Input: dimensioned drawing with shaded views. Units: mm. Origin: part minimum x, y, z. A direction names the side the tool comes from. Round coordinates to 2 decimals unless told otherwise and drop trailing zeros. Loops run counter-clockwise (first coordinate to the right, second up) from the corner with the lowest first, then second, coordinate; pieces in that order, holes last. Notation, with made-up numbers: (-8, -7.75) - (3, -7.75) arc R12 ccw to (3, -3.75) - close; hole circle Ø3 at (40.25, -34). An arc over 180 degrees is marked (long way). One line per question, with ' | ' between items. Start each with the question number.
Item 1: Section D-D, the plane z = 86. Return loops of the section in (x, y).
Item 2: First-contact query: pin 1 (12 mm diameter, centred on y = 122, z = 266, fed in from -X); pin 2 (3 mm diameter, centred on x = 233.5, z = 801.5, fed in from -Y); pin 3 (10 mm diameter, centred on x = 418, z = 441.5, fed in from +Y). Flat tips, straight axial feed; report the tip coordinate or a pass-through.
Item 3: Section B-B, the plane z = 562. Return loops of the section in (x, y).
Item 4: Section C-C, the plane x = 327.5. Return loops of the section in (y, z), plus the area to 3 significant figures.
Item 5: Material intervals for line 1 along Z through (x, y) = (676, 86); line 2 along Y through (x, z) = (394, 626.5); line 3 along Y through (x, z) = (71.5, 714), sorted ascending.
Item 6: Section A-A, the plane y = 75. Return loops of the section in (x, z), plus the area to 3 significant figures.
Item 7: Set-up query: the marked faces 1, 2 and 3. Return all of +Z, -Z, +X, -X, +Y, -Y with unobstructed straight access to the full face (end or side cutting, diameter ignored); none if empty.
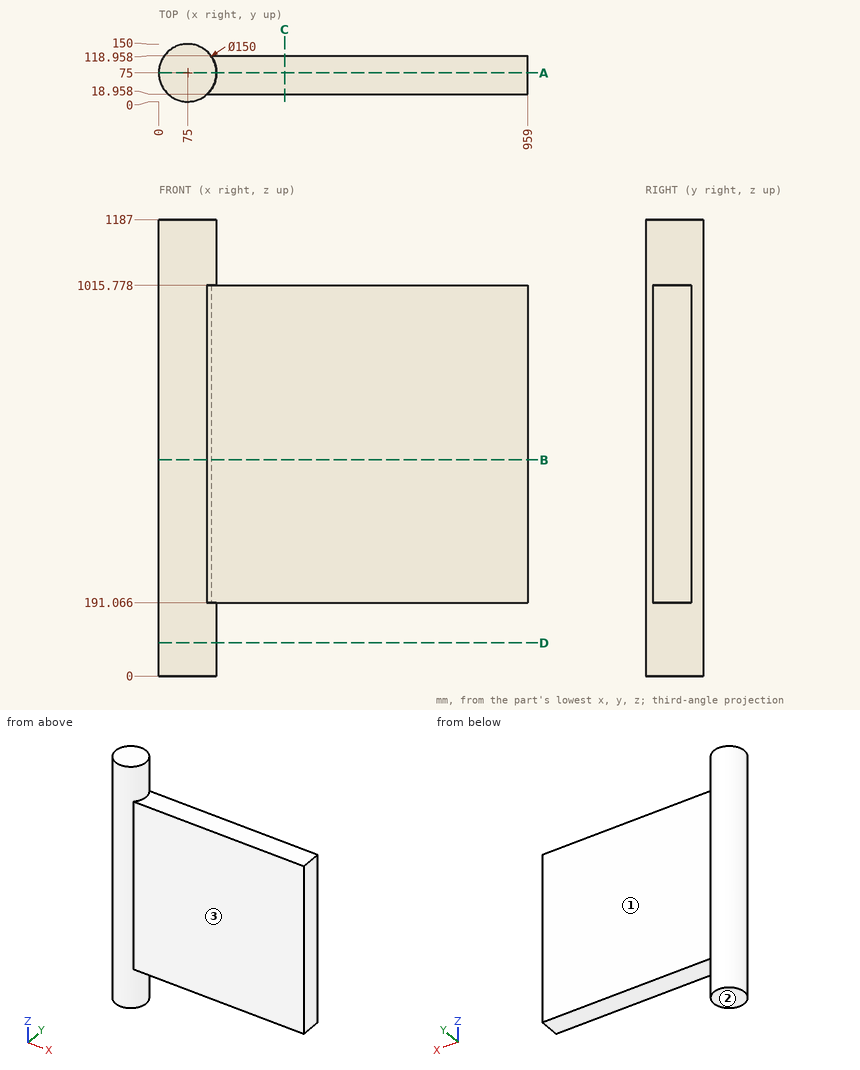
Return value:
1) outline: circle Ø150 at (75, 75)
2) pin 1: x = 12.2 | pin 2: y = 18.96 | pin 3: y = 118.96
3) outline: (124.84, 18.96) - (959, 18.96) - (959, 118.96) - (135.77, 118.96) arc R75 ccw (long way) to start
4) outline: (18.96, 191.07) - (118.96, 191.07) - (118.96, 1015.78) - (18.96, 1015.78) - close | area: 82,500 mm2
5) line 1: 191.07 to 1015.78 | line 2: 18.96 to 118.96 | line 3: 0.08 to 149.92
6) outline: (0, 0) - (150, 0) - (150, 191.07) - (959, 191.07) - (959, 1015.78) - (150, 1015.78) - (150, 1187) - (0, 1187) - close | area: 845,000 mm2
7) face 1: +Z, -Z, +X, +Y | face 2: -Z, +X, -X, +Y, -Y | face 3: +Z, -Z, +X, -Y
